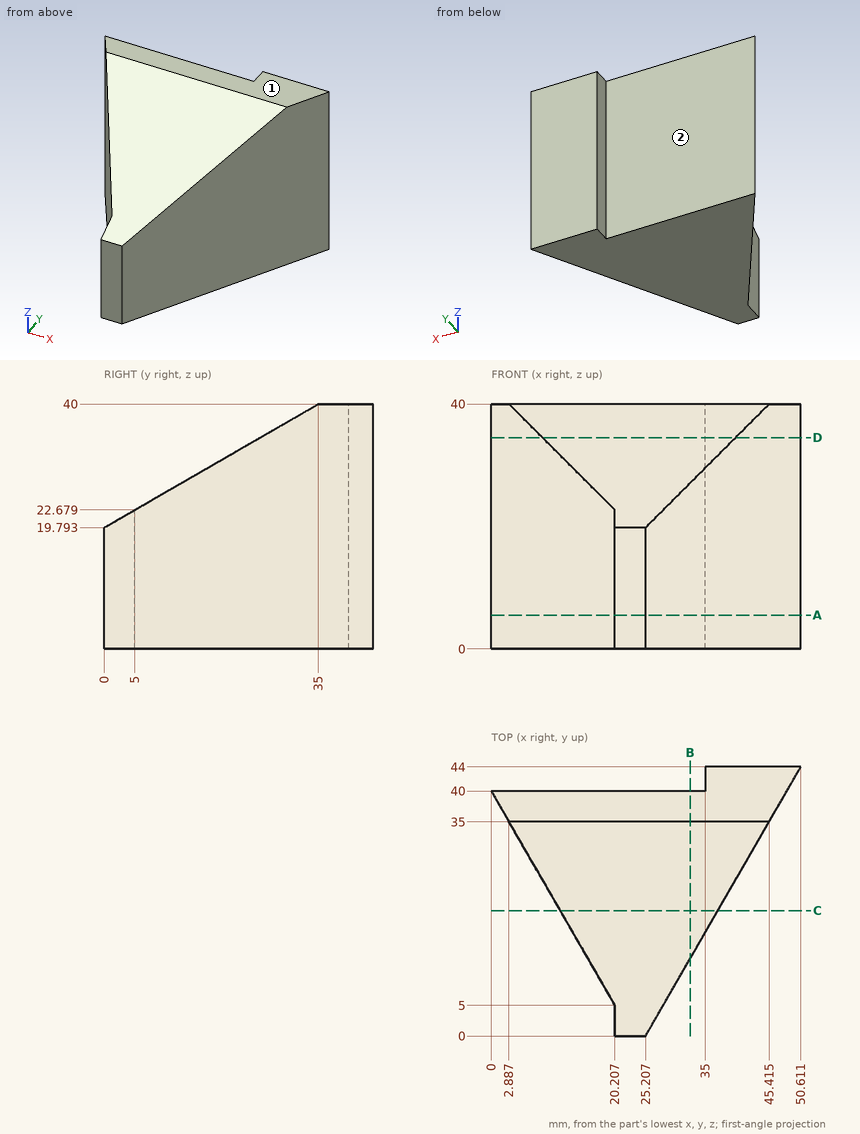
The figure shows three views and two pictorial views of one solid part (mm, origin at its lowest corner). Answer the questions. A direction names the side the tool comes from. Give positions to 0.01 mm unless a question says otherwise; leave off trailing zeros. Loops run counter-clockwise (first coordinate to the right, second up) from the corner with the lowest first, then second, coordinate; pieces in that order, holes last. Notation, with made-up numbers: (16.25, -31.75) -> (47.25, -31.75) arc R13 ccw to (47.25, -19.75) -> close; hole circle Ø11 at (-18.75, 26.5). An arc over 180 degrees is marked (long way). Put each result on its own line as item: value. Start each with the question number.
Item 1: The part is cut by section C-C (y = 20.5). Give the vertices of the cut face in (x, z).
Item 2: Each of these flat-tipped pins is pushed along its axis until it touches: P1, Ø3, axis at y = 43, z = 16, coming from the -X side; P2, Ø1, axis at y = 14, z = 9, coming from the +X side; P3, Ø1, axis at x = 32.5, z = 10.5, coming from the +Y side. Where does it stop, or does it pass through?
Item 3: The part is cut by section B-B (x = 32.5). Give the vertices of the cut face in (y, z) (1 decimal).
Item 4: Which of the six approach directions +Z, -Z, +X, -X, +Y, -Y give full straight-line access (tool end or side, diameter ignored) to the marked faces 1 and 2?
Item 5: Find the intervals of material crossed by L1, parallel to X at y = 35, z = 7.5 (1 decimal); L2, parallel to Y at x = 22, z = 7.5; L3, parallel to X at y = 33, z = 27, in increasing order. Write a range as [from, to].
Item 6: The part is cut by section A-A (z = 5.5). Give the vertices of the cut face in (x, y).
Item 7: The part is cut by section D-D (z = 34.5). Give the vertices of the cut face in (x, y) (1 decimal).
Answers below:
1. outline: (11.26, 0) -> (37.04, 0) -> (37.04, 31.63) -> (11.26, 31.63) -> close
2. P1: x = 35
2. P2: x = 33.58
2. P3: y = 40
3. outline: (12.6, 0) -> (40, 0) -> (40, 40) -> (35, 40) -> (12.6, 27.1) -> close
4. face 1: +Z, +X, -X, +Y, -Y
4. face 2: +Z, -Z, -X, +Y
5. L1: [2.9, 45.4]
5. L2: [0, 40]
5. L3: [4.04, 44.26]
6. outline: (0, 40) -> (20.21, 5) -> (20.21, 0) -> (25.21, 0) -> (50.61, 44) -> (35, 44) -> (35, 40) -> close
7. outline: (0, 40) -> (8.4, 25.5) -> (39.9, 25.5) -> (50.6, 44) -> (35, 44) -> (35, 40) -> close
